Check sheet for the modelled part. Datum: model origin and axes. Units: mm. A direction names the side the tool comes from. Round coordinates to 2 decimals unless told otherwise and drop trailing zeros. Loops run counter-clockwise (first coordinate to the right, second up) from the corner with the lowest first, then second, coordinate; pieces in that order, holes last. Notation, with made-up numbers: (-39.75, -0.75) -> (-6.75, -0.75) arc R22 cw to (-6.75, 15.25) -> close; hole circle Ø4 at (73.5, 62.25). An arc over 180 degrees is marked (long way). Use one line per item in the form item = value. Start each with the question number.
(1) Draft check along Y on faces 3 (the cylindrical face through (14.591, -18.707, -2.972)), 4 (the flat face through (-10.85, -33.61, 23.85)), 5 (the cylindrical face through (-16.818, 14.426, -2.972)), 6 (the flat face through (-32, 0, 5)). Enter one of: released by +Y, released by -Y, zero draft, split by the parting line, or undercut.
(2) Set-up check for faces 1 (the flat face through (-15, -20, -1)), 2 (the flat face through (-7, 0, -5)): record each of +Z, -Z, +X, -X, +Y, -Y from which the full face is reachable in a straight line by a thin tool's end or side.
(3) Sectioned sample at D-D (z = 22). Record the cut outline in (x, y).
(4) Material ranges on probe 1 along Z at (x, y) = (-25, 0); probe 2 along Y at (x, z) = (0, 2); probe 3 along Y at (x, z) = (1, 25.5), recorded low to high. Write a range as [from, to].
(5) Sectioned sample at C-C (y = -4.5). Record the cut outline in (x, z), and give its area (3 significant figures).
(6) Sectioned sample at B-B (z = 13.5). Record the cut outline in (x, y), and give its area (3 significant figures).
(7) Sectioned sample at A-A (z = 33). Record the cut outline in (x, y), and give its area (3 significant figures).
(8) Go/stop test with flat-tipped pins: pin 1 (6 mm diameter, centred on x = -4, z = 30.5, fed in from +Y); pin 2 (8 mm diameter, centred on x = -11, z = 33, fed in from +Y); pin 3 (1 mm diameter, centred on x = -25, z = 17.5, fed in from -Y). Record where each tip stops, or that it passes through.
from build123d import *
from build123d.topology import SkipClean

# Parameters (mm, degrees)
CROQUIS1_R                   = 35.5
CROQUIS1_R_2                 = 3.25
CROQUIS1_R_3                 = 3.15
SALIENTE_EXTRUIR1_DEPTH      = 5
SALIENTE_EXTRUIR2_DEPTH      = 35
CROQUIS3_R                   = 6
CORTAR_EXTRUIR1_DEPTH        = 85.042735149
CORTAR_EXTRUIR2_REACH        = 66.191
CORTAR_EXTRUIR2_END_RADIUS   = 6
CROQUIS4_R                   = 1.5
CORTAR_EXTRUIR_L_MINA1_START = 11
CORTAR_EXTRUIR_L_MINA1_DEPTH = 13
CORTAR_EXTRUIR3_REACH        = 94.695
CORTAR_EXTRUIR3_END_RADIUS   = 20
CROQUIS6_R                   = 2
CORTAR_EXTRUIR_L_MINA2_START = 10
CORTAR_EXTRUIR_L_MINA2_DEPTH = 13
CROQUIS10_R                  = 35.5
CROQUIS10_R_2                = 3.25
CROQUIS10_R_3                = 3.15
SALIENTE_EXTRUIR4_DEPTH      = 5
CROQUIS8_R                   = 5.25
CORTAR_EXTRUIR4_DEPTH        = 6


with BuildPart() as part:
    # Croquis1 → Saliente-Extruir1 (new body)
    with BuildSketch(Plane.XY):
        Circle(CROQUIS1_R)
        Circle(CROQUIS1_R_2, mode=Mode.SUBTRACT)
        with Locations((17.500892834, 17.500892834)):
            Circle(CROQUIS1_R_3, mode=Mode.SUBTRACT)
        with Locations((17.500892834, -17.500892834)):
            Circle(CROQUIS1_R_3, mode=Mode.SUBTRACT)
        with Locations((-17.500892834, -17.500892834)):
            Circle(CROQUIS1_R_3, mode=Mode.SUBTRACT)
        with Locations((-17.500892834, 17.500892834)):
            Circle(CROQUIS1_R_3, mode=Mode.SUBTRACT)
    extrude(amount=SALIENTE_EXTRUIR1_DEPTH)

    # Croquis2 → Saliente-Extruir2 (add)
    with BuildSketch(Plane.XY.offset(5)):
        with BuildLine():
            ThreePointArc((-29.330018752, -20), (35.5, 0), (-29.330018752, 20))
            Line((-29.330018752, 20), (-29.330018752, -20))
        make_face()
        with BuildLine():
            ThreePointArc((10.003105755, 17.318714596), (17.409796995, 25.000339584), (25.000892834, 17.500892834))
            ThreePointArc((25.000892834, 17.500892834), (22.739388001, 12.133568697), (17.318714596, 10.003105755))
            ThreePointArc((17.318714596, 10.003105755), (19.318052333, 5.178112981), (20, 0))
            ThreePointArc((20, 0), (19.318052333, -5.178112981), (17.318714596, -10.003105755))
            ThreePointArc((17.318714596, -10.003105755), (22.739388001, -12.133568697), (25.000892834, -17.500892834))
            ThreePointArc((25.000892834, -17.500892834), (17.409796995, -25.000339584), (10.003105755, -17.318714596))
            ThreePointArc((10.003105755, -17.318714596), (0, -20), (-10.003105755, -17.318714596))
            ThreePointArc((-10.003105755, -17.318714596), (-10.001446085, -17.409796995), (-10.000892834, -17.500892834))
            ThreePointArc((-10.000892834, -17.500892834), (-22.868216972, -22.739388001), (-17.318714596, -10.003105755))
            ThreePointArc((-17.318714596, -10.003105755), (-20, 0), (-17.318714596, 10.003105755))
            ThreePointArc((-17.318714596, 10.003105755), (-22.868216972, 22.739388001), (-10.000892834, 17.500892834))
            ThreePointArc((-10.000892834, 17.500892834), (-10.001446085, 17.409796995), (-10.003105755, 17.318714596))
            ThreePointArc((-10.003105755, 17.318714596), (0, 20), (10.003105755, 17.318714596))
        make_face(mode=Mode.SUBTRACT)
    extrude(amount=SALIENTE_EXTRUIR2_DEPTH)

    # Croquis3 → Cortar-Extruir1 (cut, through all)
    with SkipClean():  # the faces are left unmerged after this step: merging them gives an invalid solid
        with BuildSketch(Plane.ZY.offset(29.330018752)):
            with Locations((22, 0)):
                Circle(CROQUIS3_R)
        extrude(amount=-CORTAR_EXTRUIR1_DEPTH, mode=Mode.SUBTRACT)

    # Cortar-Extruir2: up to this cylinder (the profile starts outside it)
    with SkipClean():  # the faces are left unmerged after this step: merging them gives an invalid solid
        cortar_extruir2_end = Plane(origin=(27.5, 0, 22), z_dir=(-1, 0, 0)) * Cylinder(CORTAR_EXTRUIR2_END_RADIUS, 145.382, mode=Mode.PRIVATE)
        # Croquis4 → Cortar-Extruir2 (cut, up to the surface)
        with BuildSketch(Plane.XY.offset(40), mode=Mode.PRIVATE) as cortar_extruir2_sk1:
            with Locations((27.5, 0)):
                Circle(CROQUIS4_R)
        cortar_extruir2_tool1 = extrude(cortar_extruir2_sk1.sketch, amount=-CORTAR_EXTRUIR2_REACH, mode=Mode.PRIVATE) - cortar_extruir2_end
        add(cortar_extruir2_tool1.solids().sort_by_distance((27.5, 0, 40))[0], mode=Mode.SUBTRACT)

    # Croquis5 → Cortar-Extruir-Lámina1 (cut)
    with SkipClean():  # the faces are left unmerged after this step: merging them gives an invalid solid
        with BuildSketch(Plane.XY.offset(5).offset(CORTAR_EXTRUIR_L_MINA1_START)):
            Polygon((-16.202076443, -31.58706569), (-8.717795145, -34.41293431), (-9.4242623, -36.284004634), (-16.908543598, -33.458136015), align=None)
        extrude(amount=CORTAR_EXTRUIR_L_MINA1_DEPTH, mode=Mode.SUBTRACT)

    # Cortar-Extruir3: up to this cylinder (the profile starts outside it)
    with SkipClean():  # the faces are left unmerged after this step: merging them gives an invalid solid
        cortar_extruir3_end = Plane(origin=(0, 0, 22), z_dir=(0, 0, -1)) * Cylinder(CORTAR_EXTRUIR3_END_RADIUS, 230.39, mode=Mode.PRIVATE)
        # Croquis6 → Cortar-Extruir3 (cut, up to the surface)
        with BuildSketch(Plane(origin=(-12.459935794, -33, 0), x_dir=(0.935535162237637, -0.3532335774200951, 0), z_dir=(-0.35323357742009515, -0.9355351622376371, 0)), mode=Mode.PRIVATE) as cortar_extruir3_sk1:
            with Locations((0, 22)):
                Circle(CROQUIS6_R)
        cortar_extruir3_tool1 = extrude(cortar_extruir3_sk1.sketch, amount=-CORTAR_EXTRUIR3_REACH, mode=Mode.PRIVATE) - cortar_extruir3_end
        add(cortar_extruir3_tool1.solids().sort_by_distance((-12.459936, -33, 22))[0], mode=Mode.SUBTRACT)

    # Croquis7 → Cortar-Extruir-Lámina2 (cut)
    with SkipClean():  # the faces are left unmerged after this step: merging them gives an invalid solid
        with BuildSketch(Plane.XY.offset(5).offset(CORTAR_EXTRUIR_L_MINA2_START)):
            Polygon((-10.903572782, -17.554038257), (-3.419291484, -20.379906876), (-2.712824329, -18.508836552), (-10.197105627, -15.682967932), align=None)
        extrude(amount=CORTAR_EXTRUIR_L_MINA2_DEPTH, mode=Mode.SUBTRACT)

    # Croquis10 → Saliente-Extruir4 (add)
    with SkipClean():  # the faces are left unmerged after this step: merging them gives an invalid solid
        with BuildSketch(Plane(origin=(0, 0, 0), x_dir=(-1, 0, 0), z_dir=(0, 0, -1))):
            Circle(CROQUIS10_R)
            Circle(CROQUIS10_R_2, mode=Mode.SUBTRACT)
            with Locations((-17.500892834, -17.500892834)):
                Circle(CROQUIS10_R_3, mode=Mode.SUBTRACT)
            with Locations((17.500892834, 17.500892834)):
                Circle(CROQUIS10_R_3, mode=Mode.SUBTRACT)
            with Locations((17.500892834, -17.500892834)):
                Circle(CROQUIS10_R_3, mode=Mode.SUBTRACT)
            with Locations((-17.500892834, 17.500892834)):
                Circle(CROQUIS10_R_3, mode=Mode.SUBTRACT)
        extrude(amount=SALIENTE_EXTRUIR4_DEPTH)

    # Croquis8 → Cortar-Extruir4 (cut)
    with SkipClean():  # the faces are left unmerged after this step: merging them gives an invalid solid
        with BuildSketch(Plane.XY.offset(5)):
            with Locations((-17.500892834, -17.500892834)):
                Circle(CROQUIS8_R)
            with Locations((-17.500892834, 17.500892834)):
                Circle(CROQUIS8_R)
            with Locations((17.500892834, 17.500892834)):
                Circle(CROQUIS8_R)
            with Locations((17.500892834, -17.500892834)):
                Circle(CROQUIS8_R)
        extrude(amount=-CORTAR_EXTRUIR4_DEPTH, mode=Mode.SUBTRACT)


solid = part.part
Checks:
q1.face_3 = undercut
q1.face_4 = released by -Y
q1.face_5 = undercut
q1.face_6 = zero draft
q2.face_1 = +Z
q2.face_2 = -Z, +X, -X, +Y, -Y
q3.outline = (-29.33, -20) arc R35.5 ccw to (-16.2, -31.59) -> (-14.33, -32.29) -> (-9.03, -18.26) -> (-10.01, -17.89) arc R7.5 cw (long way) to (-17.32, -10) arc R20 cw to (-19.08, -6) -> (-29.33, -6) -> close; (-29.33, 6) -> (-19.08, 6) arc R20 cw to (-17.32, 10) arc R7.5 cw (long way) to (-10, 17.5) arc R7.5 cw to (-10, 17.32) arc R20 cw to (10, 17.32) arc R7.5 cw (long way) to (17.32, 10) arc R20 cw to (19.08, 6) -> (34.99, 6) arc R35.5 ccw to (-29.33, 20) -> close; (-10.59, -33.71) -> (-8.72, -34.41) arc R35.5 ccw to (34.99, -6) -> (19.08, -6) arc R20 cw to (17.32, -10) arc R7.5 cw (long way) to (10, -17.32) arc R20 cw to (-3.18, -19.75) -> (-3.42, -20.38) -> (-5.29, -19.67) -> close
q4.probe_1 = [-5, 16], [28, 40]
q4.probe_2 = [-35.5, -3.25], [3.25, 35.5]
q4.probe_3 = [-35.49, -19.97], [19.97, 35.49]
q5.outline = (-35.21, -5) -> (35.21, -5) -> (35.21, 18.03) -> (19.49, 18.03) -> (19.49, 5) -> (-19.49, 5) -> (-19.49, 18.03) -> (-29.33, 18.03) -> (-29.33, 5) -> (-35.21, 5) -> close; (-29.33, 25.97) -> (-19.49, 25.97) -> (-19.49, 40) -> (-29.33, 40) -> close; (19.49, 25.97) -> (35.21, 25.97) -> (35.21, 40) -> (19.49, 40) -> close
q5.area = 1,400 mm2
q6.outline = (-29.33, -20) arc R35.5 ccw (long way) to (-29.33, 20) -> close; hole (-17.32, -10) arc R7.5 ccw (long way) to (-10, -17.5) arc R7.5 ccw to (-10, -17.32) arc R20 ccw to (10, -17.32) arc R7.5 ccw (long way) to (17.32, -10) arc R20 ccw to (17.32, 10) arc R7.5 ccw (long way) to (10, 17.32) arc R20 ccw to (-10, 17.32) arc R7.5 ccw to (-10, 17.5) arc R7.5 ccw (long way) to (-17.32, 10) arc R20 ccw to start
q6.area = 1,910 mm2
q7.outline = (-29.33, -20) arc R35.5 ccw (long way) to (-29.33, 20) -> close; hole (-17.32, -10) arc R7.5 ccw (long way) to (-10, -17.5) arc R7.5 ccw to (-10, -17.32) arc R20 ccw to (10, -17.32) arc R7.5 ccw (long way) to (17.32, -10) arc R20 ccw to (17.32, 10) arc R7.5 ccw (long way) to (10, 17.32) arc R20 ccw to (-10, 17.32) arc R7.5 ccw to (-10, 17.5) arc R7.5 ccw (long way) to (-17.32, 10) arc R20 ccw to start; hole circle Ø3 at (27.5, 0)
q7.area = 1,900 mm2
q8.pin_1 = 35.49
q8.pin_2 = 34.8
q8.pin_3 = -25.69
